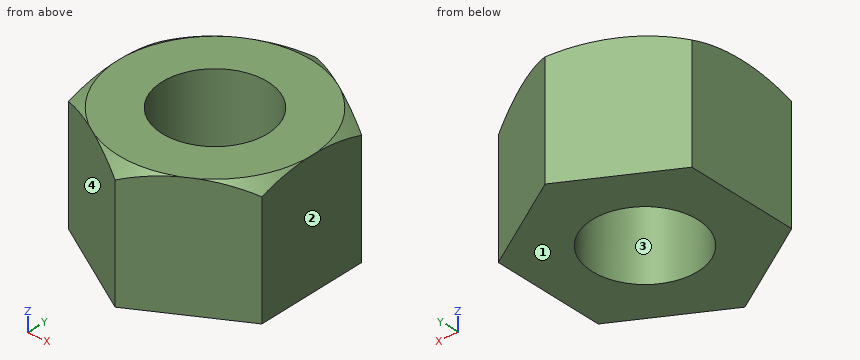
```python
from build123d import *

# Parameters (mm, degrees)
SKETCH_1_R      = 1.5
EXTRUDE_1_DEPTH = 3.5


with BuildPart() as part:
    # ｽｹｯﾁ1 → ﾎﾞｽ - 押し出し1 (new body)
    with BuildSketch(Plane.XY):
        Polygon((0, 3.175426481), (-2.75, 1.58771324), (-2.75, -1.58771324), (0, -3.175426481), (2.75, -1.58771324), (2.75, 1.58771324), align=None)
        Circle(SKETCH_1_R, mode=Mode.SUBTRACT)
    extrude(amount=EXTRUDE_1_DEPTH)

    # ｽｹｯﾁ5 → ｶｯﾄ - 回転2 (revolve, cut)
    with BuildSketch(Plane(origin=(0, 0, 0), x_dir=(0, 0, -1), z_dir=(1, 0, 0))):
        with BuildLine():
            Line((-3.227591474, 3.175426481), (-3.5, 3.175426481))
            Line((-3.5, 3.175426481), (-3.5, 2.75))
            ThreePointArc((-3.5, 2.75), (-3.368682669, 2.965842434), (-3.227591474, 3.175426481))
        make_face()
    revolve(axis=Axis((0, 0, 0), (0, 0, 1)), mode=Mode.SUBTRACT)


solid = part.part
```
Geometry: final body of the model. Coordinates: model frame, mm. Face numbers are marked on the shaded views. Coordinates: 2 decimals unless noted, no trailing zeros. Write each loop counter-clockwise with the first axis right and the second up, starting at its lowest first coordinate (ties: lowest second). Pieces come first, ordered by that corner, then holes. Notation, with made-up numbers: M 76.5,-19 L 118.5,-19 A19 cw 118.5,7 Z; hole C 59.25,66.5 d7. An arc over 180 degrees is marked long. Use CSV: the item, a comma, the result in double quotes. Start each with the question number.
1. Mould query, pull axis X, two halves, no side actions, for the marked faces 1, 2, 3 and 4. Classes: pulls with the +X half, pulls with the -X half, needs draft (parallel to the pull), parting line crosses it, or undercut.
2. First-contact query: P1, Ø1, axis at x = 1.5, z = 1, coming from the +Y side; P2, Ø1.5, axis at x = -1.5, z = 2, coming from the -Y side; P3, Ø2, axis at x = 0.5, z = 1.5, coming from the +Y side. Flat tips, straight axial feed; report the tip coordinate or a pass-through.
3. Ray query, probe 1 along X at (y, z) = (0.75, 3); probe 2 along Y at (x, z) = (-0.6, 1.75); probe 3 along Y at (x, z) = (0.25, 0.65). Return the intervals inside material, ascending.
4. Cut plane A-A on z = 0.3. Return the cut outline in (x, y).
Entries:
1,face 1,"needs draft"
1,face 2,"pulls with the +X half"
1,face 3,"undercut"
1,face 4,"pulls with the -X half"
2,P1,"y = 2.6"
2,P2,"y = -2.74"
2,P3,"y = 3.18"
3,probe 1,"-2.75 to -1.3, 1.3 to 2.75"
3,probe 2,"-2.83 to -1.37, 1.37 to 2.83"
3,probe 3,"-3.03 to -1.48, 1.48 to 3.03"
4,outline,"M -2.75,-1.59 L 0,-3.18 L 2.75,-1.59 L 2.75,1.59 L 0,3.18 L -2.75,1.59 Z; hole C 0,0 d3"
